The listing builds one solid part. Answer for the finished solid, in the listing's coordinates (mm). A direction names the side the tool comes from. Round coordinates to 2 decimals unless told otherwise and drop trailing zeros. Write each loop counter-clockwise with the first axis right and the second up, starting at its lowest first coordinate (ties: lowest second). Pieces come first, ordered by that corner, then holes. Notation, with made-up numbers: (65, -35) - (80, -35) arc R23 ccw to (80, -17) - close; hole circle Ø5 at (43.25, 28). An arc over 180 degrees is marked (long way). Answer in a Markdown table with one row per item.
from build123d import *

# Parameters (mm, degrees)
F1_DEPTH  = 2.5
F2_T      = -2
F5_SIZE   = 1
F6_W      = 73.7499899587
F6_H      = 5
F7_DEPTH  = 37.501
F8_W      = 2
F8_H      = 7.4062455549
F9_DEPTH  = 6
F12_R     = 5
F13_DEPTH = 5
F15_D     = 6


with BuildPart() as f1:
    # F0 (on Front) → F1 (new body, symmetric)
    with BuildSketch(Plane.XZ):
        with BuildLine():
            Line((0, 10), (0, 0))
            Line((0, 0), (70, 0))
            Line((70, 0), (70, 10))
            Line((70, 10), (50, 10))
            ThreePointArc((50, 10), (46.4644660941, 11.4644660941), (45, 15))
            Line((45, 15), (45, 25))
            Line((45, 25), (35, 25))
            Line((35, 25), (35, 15))
            ThreePointArc((35, 15), (33.5355339059, 11.4644660941), (30, 10))
            Line((30, 10), (0, 10))
        make_face()
    extrude(amount=F1_DEPTH, both=True)

    # F2
    f2_openings = [f1.faces().sort_by_distance(p)[0] for p in [
        (35.933685, -2.5, 7.254637),
    ]]
    offset(amount=F2_T, openings=f2_openings)

    # F3 (on Front) → F4 (revolve)
    with BuildSketch(Plane.XZ):
        Polygon((37, 25), (40, 25), (40, 37.5), (37, 37.5), (37, 35.5), (37.5, 35.5), (37.5, 29), (37, 29), align=None)
    revolve(axis=Axis((40, 0, 31.25), (0, 0, 1)))

    # F5
    f5_edges = [f1.edges().sort_by_distance(p)[0] for p in [
        (43, 0, 37.5),
    ]]
    chamfer(f5_edges, length=F5_SIZE)

    # F6 (on face) → F7 (intersect, through all)
    with BuildSketch(Plane.XY.offset(37.5)):
        with Locations((35.0708486512, 0)):
            Rectangle(F6_W, F6_H)
    extrude(amount=-F7_DEPTH, mode=Mode.INTERSECT)

    # F8 (on face) → F9 (cut)
    with BuildSketch(Plane.XY.offset(37.5)):
        with Locations((40, -0.1854714938)):
            Rectangle(F8_W, F8_H)
    extrude(amount=-F9_DEPTH, mode=Mode.SUBTRACT)

    # F10: F1 across plane


with BuildPart() as f1_1:
    add(f1.part)
    add(f1.part.mirror(Plane.XY))

    # F11: F1 across plane


with BuildPart() as f1_2:
    add(f1_1.part)
    add(f1_1.part.mirror(Plane.YZ))

    # F12 (on face) → F13 (join, through all)
    with BuildSketch(Plane.XZ.offset(2.5)):
        with Locations((-40, 0)):
            Circle(F12_R)
        with Locations((-15, 0)):
            Circle(F12_R)
    extrude(amount=-F13_DEPTH)

    # F15 (through all)
    with Locations(Plane.XZ.offset(2.5)):
        with Locations((-40, 0), (-15, 0)):
            Hole(F15_D / 2)


solid = f1_2.part
(1) Section C-C (x = 32.5) is taken. Give the vertices of the cut face in (y, z), and give its area (3 significant figures).
Checked values:
| item | result |
|---|---|
| outline | (-2.5, -10.67) - (2.5, -10.67) - (2.5, 10.67) - (-2.5, 10.67) - (-2.5, 8.46) - (0.5, 8.46) - (0.5, 2) - (-2.5, 2) - (-2.5, -2) - (0.5, -2) - (0.5, -8.46) - (-2.5, -8.46) - close |
| area | 67.9 mm2 |
(2) For a pull along X with two mould halves and no side action, classify faces 5 (the flat face through (-42.7, -0.2, -29)), 6 (the flat face through (41, 0, 35)), 7 (the flat face through (68, -1, -5)), 8 (the cylindrical face through (47, 0, -11)) as pulls with the +X half, pulls with the -X half, needs draft (parallel to the pull), parting line crosses it, or undercut.
Checked values:
| item | result |
|---|---|
| face 5 | needs draft |
| face 6 | undercut |
| face 7 | undercut |
| face 8 | pulls with the +X half |
(3) Section A-A (z = 0) is taken. Give the vertices of the cut face in (x, y), and give its area (3 significant figures).
Checked values:
| item | result |
|---|---|
| outline | (-70, -2.5) - (-43, -2.5) - (-43, 2.5) - (-70, 2.5) - close; (-37, -2.5) - (-18, -2.5) - (-18, 2.5) - (-37, 2.5) - close; (-12, -2.5) - (70, -2.5) - (70, 2.5) - (-12, 2.5) - close |
| area | 640 mm2 |
(4) Find the intervals of material crossed by line 1 (X direction, y = -0.9, z = -18); line 2 (Z direction, x = -40, y = 0.3); line 3 (Z direction, x = 23, y = 0.1), in increasing order.
Checked values:
| item | result |
|---|---|
| line 1 | x = -45 to -43, -37 to -35, 35 to 37, 43 to 45 |
| line 2 | z = -31.5 to -23, -5 to -3, 3 to 5, 23 to 31.5 |
| line 3 | z = -10 to -8, -2 to 2, 8 to 10 |
(5) Section B-B (x = -15) is taken. Give the vertices of the cut face in (y, z), and give its area (3 significant figures).
Checked values:
| item | result |
|---|---|
| outline | (-2.5, -10) - (2.5, -10) - (2.5, -3) - (-2.5, -3) - (-2.5, -5) - (0.5, -5) - (0.5, -8) - (-2.5, -8) - close; (-2.5, 3) - (2.5, 3) - (2.5, 10) - (-2.5, 10) - (-2.5, 8) - (0.5, 8) - (0.5, 5) - (-2.5, 5) - close |
| area | 52.0 mm2 |
(6) For faces 1 (the flat face through (-59, -1, -8)), 2 (the cylindrical face through (-37.69, 0.96, 32.2)), 3 (the flat face through (35, 0, -20)), 4 (the flat face through (-70, 0, 0)), determine the directions among +Z, -Z, +X, -X, +Y, -Y from which every point of the face is accessible in a straight line to the end or side of a thin tool.
Checked values:
| item | result |
|---|---|
| face 1 | -Y |
| face 2 | none |
| face 3 | -Z, +Y, -Y |
| face 4 | +Z, -Z, -X, +Y, -Y |
(7) Section D-D (x = -48) is taken. Give the vertices of the cut face in (y, z).
Checked values:
| item | result |
|---|---|
| outline | (-2.5, -10.42) - (2.5, -10.42) - (2.5, 10.42) - (-2.5, 10.42) - (-2.5, 8.29) - (0.5, 8.29) - (0.5, 2) - (-2.5, 2) - (-2.5, -2) - (0.5, -2) - (0.5, -8.29) - (-2.5, -8.29) - close |
(8) Flat-ended cylindrical pins translate along their axes: pin 1 (1 mm diameter, centred on x = 37, z = -3, fed in from -Y); pin 2 (2.5 mm diameter, centred on y = -1, z = -34, fed in from -X); pin 3 (1.5 mm diameter, centred on x = -56.5, y = -1.5, fed in from +Z). Find the tip coordinate at first contact, or state that the pin passes through.
Checked values:
| item | result |
|---|---|
| pin 1 | stops at y = 0.5 |
| pin 2 | stops at x = -42.5 |
| pin 3 | stops at z = 10 |
